from build123d import *

# Parameters (mm, degrees)
SKETCH1_W           = 42.844819815
SKETCH1_H           = 17.78
SKETCH1_R           = 0.917394869
BOSS_EXTRUDE1_DEPTH = 1.5
SKETCH2_R           = 0.5
BOSS_EXTRUDE2_DEPTH = 7.5
SKETCH3_W           = 5
SKETCH3_H           = 7
BOSS_EXTRUDE3_DEPTH = 2
FILLET1_R           = 0.75


with BuildPart() as part:
    # Sketch1 → Boss-Extrude1 (new body)
    with BuildSketch(Plane.XY):
        with Locations((-197.662982249, 61.653534283)):
            Rectangle(SKETCH1_W, SKETCH1_H)
        with Locations((-217.982982248, 69.278534283)):
            Circle(SKETCH1_R, mode=Mode.SUBTRACT)
        with Locations((-217.982982248, 54.028534283)):
            Circle(SKETCH1_R, mode=Mode.SUBTRACT)
        with Locations((-177.342982248, 54.028534283)):
            Circle(SKETCH1_R, mode=Mode.SUBTRACT)
        with Locations((-177.342982248, 69.278534283)):
            Circle(SKETCH1_R, mode=Mode.SUBTRACT)
    extrude(amount=BOSS_EXTRUDE1_DEPTH)

    # Sketch2 → Boss-Extrude2 (add)
    with BuildSketch(Plane.XY.offset(1.5)):
        with Locations((-213.982982248, 69.278534283)):
            Circle(SKETCH2_R)
        with Locations((-213.982982248, 54.028534283)):
            Circle(SKETCH2_R)
        with Locations((-211.982982248, 69.278534283)):
            Circle(SKETCH2_R)
        with Locations((-211.982982248, 54.028534283)):
            Circle(SKETCH2_R)
        with Locations((-209.982982248, 69.278534283)):
            Circle(SKETCH2_R)
        with Locations((-209.982982248, 54.028534283)):
            Circle(SKETCH2_R)
        with Locations((-207.982982248, 69.278534283)):
            Circle(SKETCH2_R)
        with Locations((-207.982982248, 54.028534283)):
            Circle(SKETCH2_R)
        with Locations((-205.982982248, 69.278534283)):
            Circle(SKETCH2_R)
        with Locations((-205.982982248, 54.028534283)):
            Circle(SKETCH2_R)
        with Locations((-203.982982248, 69.278534283)):
            Circle(SKETCH2_R)
        with Locations((-203.982982248, 54.028534283)):
            Circle(SKETCH2_R)
        with Locations((-201.982982248, 69.278534283)):
            Circle(SKETCH2_R)
        with Locations((-201.982982248, 54.028534283)):
            Circle(SKETCH2_R)
        with Locations((-199.982982248, 69.278534283)):
            Circle(SKETCH2_R)
        with Locations((-199.982982248, 54.028534283)):
            Circle(SKETCH2_R)
        with Locations((-197.982982248, 69.278534283)):
            Circle(SKETCH2_R)
        with Locations((-197.982982248, 54.028534283)):
            Circle(SKETCH2_R)
        with Locations((-195.982982248, 69.278534283)):
            Circle(SKETCH2_R)
        with Locations((-195.982982248, 54.028534283)):
            Circle(SKETCH2_R)
        with Locations((-193.982982248, 69.278534283)):
            Circle(SKETCH2_R)
        with Locations((-193.982982248, 54.028534283)):
            Circle(SKETCH2_R)
        with Locations((-191.982982248, 69.278534283)):
            Circle(SKETCH2_R)
        with Locations((-191.982982248, 54.028534283)):
            Circle(SKETCH2_R)
        with Locations((-189.982982248, 69.278534283)):
            Circle(SKETCH2_R)
        with Locations((-189.982982248, 54.028534283)):
            Circle(SKETCH2_R)
        with Locations((-187.982982248, 69.278534283)):
            Circle(SKETCH2_R)
        with Locations((-187.982982248, 54.028534283)):
            Circle(SKETCH2_R)
        with Locations((-185.982982248, 69.278534283)):
            Circle(SKETCH2_R)
        with Locations((-185.982982248, 54.028534283)):
            Circle(SKETCH2_R)
        with Locations((-183.982982248, 69.278534283)):
            Circle(SKETCH2_R)
        with Locations((-183.982982248, 54.028534283)):
            Circle(SKETCH2_R)
        with Locations((-181.982982248, 69.278534283)):
            Circle(SKETCH2_R)
        with Locations((-181.982982248, 54.028534283)):
            Circle(SKETCH2_R)
    extrude(amount=BOSS_EXTRUDE2_DEPTH)

    # Sketch3 → Boss-Extrude3 (add)
    with BuildSketch(Plane(origin=(0, 0, 0), x_dir=(-1, 0, 0), z_dir=(0, 0, -1))):
        with Locations((217.835392156, 61.653534283)):
            Rectangle(SKETCH3_W, SKETCH3_H)
    extrude(amount=BOSS_EXTRUDE3_DEPTH)

    # Fillet1
    fillet1_edges = [part.edges().sort_by_distance(p)[0] for p in [
        (-219.710392156, 58.153534283, 0),
        (-219.710392156, 65.153534283, 0),
        (-217.835392156, 58.153534283, -2),
        (-217.835392156, 65.153534283, -2),
    ]]
    fillet(fillet1_edges, radius=FILLET1_R)


solid = part.part
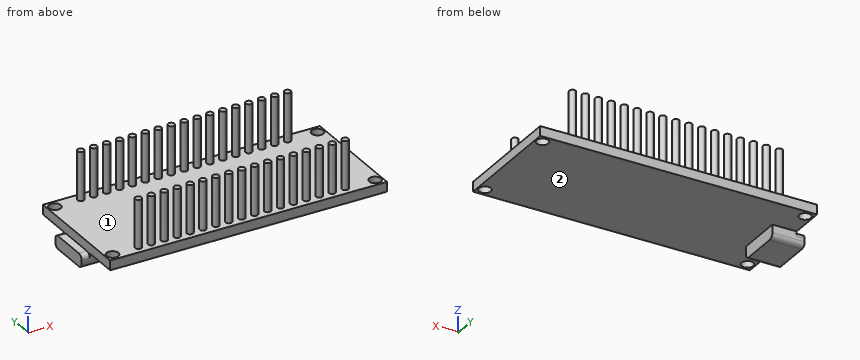
Verification items for the finished model (mm, model axes). Face numbers are marked on the shaded views. Give positions to 0.01 mm unless a question says otherwise; leave off trailing zeros. Write each loop counter-clockwise with the first axis right and the second up, starting at its lowest first coordinate (ties: lowest second). Pieces come first, ordered by that corner, then holes. Notation, with made-up numbers: M -8.5,49.25 L -2.5,49.25 A28 ccw -2.5,76.25 Z; hole C 67.25,5 d6. An arc over 180 degrees is marked long. Put each result on its own line as item: value. Start each with the question number.
1. Scan lines: line 1 along Y through (x, z) = (-184, 2.75); line 2 along X through (y, z) = (69.25, 0.25); line 3 along X through (y, z) = (69, 1.25). Record each from-to range of solid material in increasing order. Write a range as [from, to].
2. Go/stop test with flat-tipped pins: pin 1 Ø1.1 at (x, y) = (-177.34, 54.03) entering from +Z; pin 2 Ø1.4 at (x, z) = (-218.5, -1) entering from -Y; pin 3 Ø10 at (x, y) = (-208, 61.5) entering from +Z; pin 4 Ø5 at (x, y) = (-209, 67) entering from +Z. Record where each tip stops, or that it passes through.
3. Section check C-C (x = -217.5). Record the cut outline in (y, z).
4. Draft check along Y on the marked faces 1 and 2. Enter one of: +Y half, -Y half, draft (parallel to the pull), parting line (faces both ways), or undercut.
5. Section check B-B (z = 2.75). Give the number of separate pieces and of enclosed holes in the cut face, and give its area (3 significant figures).
6. Section check D-D (x = -184). Record the cut outline in (y, z), and give its area (3 significant figures).
7. Section check A-A (y = 63.25). Record the cut outline in (x, z), and give its area (3 significant figures).
Answer list:
1. line 1: [53.53, 54.53], [68.78, 69.78]
1. line 2: [-219.09, -218.9], [-217.07, -178.26], [-176.43, -176.24]
1. line 3: [-219.09, -218.86], [-217.11, -178.22], [-176.47, -176.24]
2. pin 1: through
2. pin 2: y = 58.15
2. pin 3: z = 1.5
2. pin 4: z = 9
3. outline: M 52.76,0 L 53.25,0 L 53.25,1.5 L 52.76,1.5 Z; M 54.81,0 L 58.15,0 L 58.15,-1.25 A0.75 ccw 58.9,-2 L 64.4,-2 A0.75 ccw 65.15,-1.25 L 65.15,0 L 68.5,0 L 68.5,1.5 L 54.81,1.5 Z; M 70.06,0 L 70.54,0 L 70.54,1.5 L 70.06,1.5 Z
4. face 1: undercut
4. face 2: draft
5. separate pieces: 34
5. enclosed holes: 0
5. area: 26.7 mm2
6. outline: M 52.76,0 L 70.54,0 L 70.54,1.5 L 69.78,1.5 L 69.78,9 L 68.78,9 L 68.78,1.5 L 54.53,1.5 L 54.53,9 L 53.53,9 L 53.53,1.5 L 52.76,1.5 Z
6. area: 41.7 mm2
7. outline: M -220.34,-2 L -215.34,-2 L -215.34,0 L -176.24,0 L -176.24,1.5 L -219.09,1.5 L -219.09,0 L -220.34,0 Z
7. area: 74.3 mm2
